Here's how the part is built. I have some questions about the finished solid (model axes, mm). A direction names the side the tool comes from. Coordinates: 2 decimals unless noted, no trailing zeros. Loops run counter-clockwise (first coordinate to the right, second up) from the corner with the lowest first, then second, coordinate; pieces in that order, holes last. Notation, with made-up numbers: (6.5, -28.5) - (11.5, -28.5) arc R25 cw to (11.5, 8.5) - close; hole circle Ø3 at (39.25, 61.25). An arc over 180 degrees is marked (long way). Use a Markdown table: item, result.
```python
from build123d import *

# Parameters (mm, degrees)
F1_DEPTH    = 127
F2_W        = 2.159
F2_H        = 7.62
F3_DEPTH    = 63.5
F4_T        = -2.54
F5_R        = 2.54
F6_T4_DEPTH = 20.1763121576


# Not quite as in the source:
# - a fillet or chamfer that OpenCascade refuses, or shapes differently, is made with other operations: its cross-section is extruded or revolved along the edge and cut away or added


with BuildPart() as f1:
    # F0 (on Top) → F1 (new body)
    with BuildSketch(Plane.XY):
        Polygon((-5.969, -11.7475), (5.969, -11.7475), (10.922, -6.477), (10.922, 6.477), (5.969, 11.7475), (-5.969, 11.7475), (-10.922, 6.477), (-10.922, -6.477), align=None)
    extrude(amount=F1_DEPTH)

    # F2 (on face) → F3 (cut)
    with BuildSketch(Plane.XY.offset(127)):
        Rectangle(F2_W, F2_H)
    extrude(amount=-F3_DEPTH, mode=Mode.SUBTRACT)

    # F4
    f4_openings = [f1.faces().sort_by_distance(p)[0] for p in [
        (0, 0, 0),
    ]]
    offset(amount=F4_T, openings=f4_openings, kind=Kind.INTERSECTION)

    # F5
    f5_edges = [f1.edges().sort_by_distance(p)[0] for p in [
        (10.922, 0, 127),
        (0, 11.7475, 127),
        (-10.922, 0, 127),
        (0, -11.7475, 127),
        (-8.4455, 9.11225, 127),
        (8.4455, 9.11225, 127),
        (8.4455, -9.11225, 127),
        (-8.4455, -9.11225, 127),
    ]]
    fillet(f5_edges, radius=F5_R)

    # F6: fillet of radius 2.54 on 1 edges, made by hand


with BuildPart() as f6_tool2:
    # F6_s3 → F6_t4 (new body)
    with BuildSketch(Plane.XZ.offset(10.0881560788)):
        with BuildLine():
            ThreePointArc((1.0795, 66.0112624315), (0.4655503628, 64.3553850206), (-1.0795, 63.5))
            Line((-1.0795, 63.5), (1.0795, 63.5))
            Line((1.0795, 63.5), (1.0795, 66.0112624315))
        make_face()
    extrude(amount=-F6_T4_DEPTH)

    split(bisect_by=Plane.XZ.offset(6.35), keep=Keep.BOTTOM)

    split(bisect_by=Plane.XZ.offset(-6.35), keep=Keep.TOP)


with BuildPart() as f1_1:
    add(f1.part)

    # F6_t1: union F6_tool2
    add(f6_tool2.part)


solid = f1_1.part
```
Q1. I want a section at A-A, the plane z = 75.5. Write out the boundary of the cut face in (x, y).
Check values:
| item | result |
|---|---|
| outline | (-10.92, -6.48) - (-5.97, -11.75) - (5.97, -11.75) - (10.92, -6.48) - (10.92, 6.48) - (5.97, 11.75) - (-5.97, 11.75) - (-10.92, 6.48) - close; (-3.62, -6.35) - (3.62, -6.35) - (3.62, 6.35) - (-3.62, 6.35) - close; hole (-8.38, -5.47) - (-4.87, -9.21) - (4.87, -9.21) - (8.38, -5.47) - (8.38, 5.47) - (4.87, 9.21) - (-4.87, 9.21) - (-8.38, 5.47) - close; hole (-1.08, -3.81) - (1.08, -3.81) - (1.08, 3.81) - (-1.08, 3.81) - close |
Q2. Will these pins go through, and if not, where does the flat tip stop? P1, Ø8.5, axis at x = -0.5, y = 3.5, coming from the -Z side; P2, Ø1.5, axis at y = 8, z = 30.5, coming from the +X side; P3, Ø2, axis at x = -1.5, y = -7.5, coming from the -Z side.
Check values:
| item | result |
|---|---|
| P1 | z = 60.96 |
| P2 | x = 10.2 |
| P3 | z = 124.46 |
Q3. I want a section at C-C, the plane y = 0.25. Write out the boundary of the cut face in (x, z).
Check values:
| item | result |
|---|---|
| outline | (-10.92, 0) - (-8.38, 0) - (-8.38, 124.46) - (-3.62, 124.46) - (-3.62, 60.96) - (3.62, 60.96) - (3.62, 124.46) - (8.38, 124.46) - (8.38, 0) - (10.92, 0) - (10.92, 124.46) arc R2.54 ccw to (8.38, 127) - (1.08, 127) - (1.08, 66.01) arc R2.54 cw to (-1.08, 63.5) - (-1.08, 127) - (-8.38, 127) arc R2.54 ccw to (-10.92, 124.46) - close |
Q4. I want a section at B-B, the plane z = 26. Write out the boundary of the cut face in (x, y).
Check values:
| item | result |
|---|---|
| outline | (-10.92, -6.48) - (-5.97, -11.75) - (5.97, -11.75) - (10.92, -6.48) - (10.92, 6.48) - (5.97, 11.75) - (-5.97, 11.75) - (-10.92, 6.48) - close; hole (-8.38, -5.47) - (-4.87, -9.21) - (4.87, -9.21) - (8.38, -5.47) - (8.38, 5.47) - (4.87, 9.21) - (-4.87, 9.21) - (-8.38, 5.47) - close |
Q5. Please list where these lines run through material, in increasing order: L1, parallel to X at y = 1.5, z = 109.5; L2, parallel to X at y = -4.75, z = 115.5; L3, parallel to Y at x = 2, z = 106. Write a range as from..to.
Check values:
| item | result |
|---|---|
| L1 | -10.92..-8.38, -3.62..-1.08, 1.08..3.62, 8.38..10.92 |
| L2 | -10.92..-8.38, -3.62..3.62, 8.38..10.92 |
| L3 | -11.75..-9.21, -6.35..6.35, 9.21..11.75 |
Q6. Which directions (+Z, -Z, +X, -X, +Y, -Y) give clear straight access to the entire face, cutting with the end or side of a thin tool? Please do faces 4 (the face through (-7.88, -8.65, 126.24)), 5 (the face through (-1.08, 0, 96)), 6 (the face through (0, 9.208, 61)).
Check values:
| item | result |
|---|---|
| face 4 | +Z, -X, -Y |
| face 5 | +Z |
| face 6 | -Z |
Q7. If we mould it in two halves opening along Y, with no side actions, what happens to faces 1 (the face through (0, -11.748, 61)), 2 (the face through (10.922, 0, 61)), 3 (the face through (3.62, 0, 93))? For each: pulls with the +Y half, pulls with the -Y half, needs draft (parallel to the pull), parting line crosses it, or undercut.
Check values:
| item | result |
|---|---|
| face 1 | pulls with the -Y half |
| face 2 | needs draft |
| face 3 | undercut |
